Model file for the job. Use its own axes, mm. A direction names the side the tool comes from. Round coordinates to 2 decimals unless told otherwise and drop trailing zeros. Order: outer loops, then holes, each group sorted by start corner. A loop starts at its lowest first (then second) coordinate and runs counter-clockwise, first axis right, second up. Notation, with made-up numbers: (0, 31) -> (7, 31) arc R14 ccw to (7, 54) -> close; hole circle Ø11 at (31.25, -11.5). An arc over 180 degrees is marked (long way). Put each result on its own line as item: value. Start each with the question number.
Q1. Pull direction Z, two halves, no side cores. Call faces 1 (the face through (-0.468, -11.633, 1.565)), 2 (the face through (-2.628, 0.059, 8.334)), 3 (the face through (2, -2, 10.16)): released by +Z, released by -Z, zero draft, split by the parting line, or undercut.
Q2. Cut at C-C, the plane x = -8.5. List the corners of the cut face in (y, z) (3 decimals).
Q3. Flat gauge pins, fed straight in: P1, Ø6, axis at x = 1.5, y = 4.5, coming from the -Z side; P2, Ø5, axis at y = 10, z = 3.5, coming from the -X side; P3, Ø1, axis at x = 7.5, z = 1.5, coming from the +Y side; P4, Ø3.5, axis at x = 9.525, y = 0, coming from the -Z side. Where does each tip first touch, or does it go through?
Q4. Probe L1, parallel to Y at x = 0, z = 6.25; L2, parallel to Z at x = -8.75, y = -8.75 (3 decimals). List the from-to ranges inside material, lowest first.
Q5. Cut at B-B, the plane y = 0. List the corners of the cut face in (x, z) (3 decimals).
Q6. Cut at A-A, the plane x = 0. List the corners of the cut face in (y, z) (3 decimals).
Q7. 3-axis set-ups, long thin cutter, end or side, ignore diameter. For faces 4 (the face through (3, 3, 3.175)), 5 (the face through (0, -3, 0)): which of +Z, -Z, +X, -X, +Y, -Y reach the whole face in a straight line?
from build123d import *

# Parameters (mm, degrees)
SKETCH2_R           = 12.7
SKETCH2_R_2         = 3.81
SKETCH2_R_3         = 2.159
BOSS_EXTRUDE1_DEPTH = 3.175
SKETCH2_3_R         = 3.81
SKETCH2_3_R_2       = 2
BOSS_EXTRUDE2_DEPTH = 10.16
SKETCH4_R           = 1.35
CUT_EXTRUDE1_DEPTH  = 12.7


with BuildPart() as part:
    # Sketch2 → Boss-Extrude1 (new body)
    with BuildSketch(Plane.XY):
        Circle(SKETCH2_R)
        Circle(SKETCH2_R_2, mode=Mode.SUBTRACT)
        with Locations((0, 9.525)):
            Circle(SKETCH2_R_3, mode=Mode.SUBTRACT)
        with Locations((9.525, 0)):
            Circle(SKETCH2_R_3, mode=Mode.SUBTRACT)
        with Locations((0, -9.525)):
            Circle(SKETCH2_R_3, mode=Mode.SUBTRACT)
        with Locations((-9.525, 0)):
            Circle(SKETCH2_R_3, mode=Mode.SUBTRACT)
    extrude(amount=BOSS_EXTRUDE1_DEPTH)

    # Sketch2<3> → Boss-Extrude2 (add)
    with BuildSketch(Plane.XY):
        Circle(SKETCH2_3_R)
        Circle(SKETCH2_3_R_2, mode=Mode.SUBTRACT)
    extrude(amount=BOSS_EXTRUDE2_DEPTH)

    # Sketch4 → Cut-Extrude1 (cut)
    with BuildSketch(Plane(origin=(0, 0, 0), x_dir=(0, 0, -1), z_dir=(1, 0, 0))):
        with Locations((-6.985, 0)):
            Circle(SKETCH4_R)
    extrude(amount=-CUT_EXTRUDE1_DEPTH, mode=Mode.SUBTRACT)


solid = part.part
Ans:
1. face 1: zero draft
1. face 2: undercut
1. face 3: released by +Z
2. outline: (-9.436, 0) -> (-1.9, 0) -> (-1.9, 3.175) -> (-9.436, 3.175) -> close; (1.9, 0) -> (9.436, 0) -> (9.436, 3.175) -> (1.9, 3.175) -> close
3. P1: stops at z = 0
3. P2: stops at x = -10.23
3. P3: stops at y = 10.6
3. P4: passes through
4. L1: y = -3.81 to -2, 2 to 3.81
4. L2: z = 0 to 3.175
5. outline: (-12.7, 0) -> (-11.684, 0) -> (-11.684, 3.175) -> (-12.7, 3.175) -> close; (-7.366, 0) -> (-2, 0) -> (-2, 5.635) -> (-3.81, 5.635) -> (-3.81, 3.175) -> (-7.366, 3.175) -> close; (-3.81, 8.335) -> (-2, 8.335) -> (-2, 10.16) -> (-3.81, 10.16) -> close; (2, 0) -> (7.366, 0) -> (7.366, 3.175) -> (3.81, 3.175) -> (3.81, 10.16) -> (2, 10.16) -> close; (11.684, 0) -> (12.7, 0) -> (12.7, 3.175) -> (11.684, 3.175) -> close
6. outline: (-12.7, 0) -> (-11.684, 0) -> (-11.684, 3.175) -> (-12.7, 3.175) -> close; (-7.366, 0) -> (-2, 0) -> (-2, 10.16) -> (-3.81, 10.16) -> (-3.81, 3.175) -> (-7.366, 3.175) -> close; (2, 0) -> (7.366, 0) -> (7.366, 3.175) -> (3.81, 3.175) -> (3.81, 10.16) -> (2, 10.16) -> close; (11.684, 0) -> (12.7, 0) -> (12.7, 3.175) -> (11.684, 3.175) -> close
7. face 4: +Z
7. face 5: -Z, +X, -X, +Y, -Y
